The listing builds one solid part. Answer for the finished solid, in the listing's coordinates (mm). A direction names the side the tool comes from. Coordinates: 2 decimals unless noted, no trailing zeros. Loops run counter-clockwise (first coordinate to the right, second up) from the corner with the lowest first, then second, coordinate; pieces in that order, holes last. Notation, with made-up numbers: M 68.5,-14.75 L 87.5,-14.75 A27 cw 87.5,16.25 Z; hole C 11,-22 d1. An arc over 180 degrees is marked long. Answer as a JSON object with one key per item and string values. Group by question number.
1. A cutting plane is placed at B-B on z = 0. Give the vertices of the cut face in (x, y).
2. Straight lines are drawn through the part: L1, parallel to Z at x = 38.1, y = -8; L2, parallel to X at y = -13, z = -25; L3, parallel to Z at x = -42.5, y = -12.5. For each, find the intervals that lie inside material, in ascending order.
3. Given pin 1 (1.5 mm diameter, centred on x = -7, y = -22.5, fed in from -Z); pin 2 (6 mm diameter, centred on x = -20.5, y = -39.5, fed in from -Z); pin 3 (1 mm diameter, centred on y = -52, z = -3, fed in from +X); pin 4 (11.5 mm diameter, centred on x = -38.1, z = -25.4, fed in from -Y), each flat-ended and moving along its own axis, determine where each tip first touches the part or whether it passes through.
4. A cutting plane is placed at C-C on y = -12.5. Give the vertices of the cut face in (x, z), and give its area (3 significant figures).
5. Determine the mould class of faces 1 (the face through (-5.506, -26.871, 24.796)), 2 (the face through (33.06, -10.43, -29.26)), 3 (the face through (0, -58.674, 0)) for opening direction X: released by +X, released by -X, zero draft, split by the parting line, or undercut.
6. A cutting plane is placed at D-D on x = 0. Give the vertices of the cut face in (y, z).
7. For faces 4 (the face through (31, -20.574, 0)), 5 (the face through (17, -33.274, 9)), 6 (the face through (-32.234, -10.431, 22.968)), determine the directions among +Z, -Z, +X, -X, +Y, -Y from which every point of the face is accessible in a straight line to the end or side of a thin tool.
8. A cutting plane is placed at A-A on x = 38.1. Give the vertices of the cut face in (y, z).
from build123d import *

# Parameters (mm, degrees)
F0_W     = 101.6
F0_H     = 76.2
F1_DEPTH = 20.574
F2_R     = 6.35
F3_DEPTH = 25.4
F4_W     = 25.4
F4_H     = 38.1
F6_W     = 6.35
F6_H     = 14.2712268918
F8_SIZE  = 2.54
F9_R     = 2.54
F10_R    = 2.54


with BuildPart() as f1:
    # F0 (on Front) → F1 (new body)
    with BuildSketch(Plane.XZ):
        Rectangle(F0_W, F0_H)
    extrude(amount=F1_DEPTH)

    # F2 (on face) → F3 (cut)
    with BuildSketch(Plane.XZ.offset(20.574)):
        with Locations((38.1, -25.4)):
            Circle(F2_R)
        with Locations((-38.1, -25.4)):
            Circle(F2_R)
        with Locations((-38.1, 25.4)):
            Circle(F2_R)
        with Locations((38.1, 25.4)):
            Circle(F2_R)
    extrude(amount=-F3_DEPTH, mode=Mode.SUBTRACT)

    # F4 (on Top) → F5 (revolve)
    with BuildSketch(Plane.XY):
        with Locations((12.7, -39.624)):
            Rectangle(F4_W, F4_H)
    revolve(axis=Axis((0, -39.624, 0), (0, 1, 0)))

    # F6 (on Right) → F7 (revolve, cut)
    with BuildSketch(Plane.YZ):
        with Locations((-36.449, 26.1856134459)):
            Rectangle(F6_W, F6_H)
    revolve(axis=Axis((0, -58.674, 0), (0, 1, 0)), mode=Mode.SUBTRACT)

    # F8
    f8_edges = [f1.edges().sort_by_distance(p)[0] for p in [
        (0, -20.574, 38.1),
        (50.8, -20.574, 0),
        (0, -20.574, -38.1),
        (-50.8, -20.574, 0),
    ]]
    chamfer(f8_edges, length=F8_SIZE)

    # F9
    f9_edges = [f1.edges().sort_by_distance(p)[0] for p in [
        (-25.4, -20.574, 0),
        (-25.4, -33.274, 0),
        (-25.4, -39.624, 0),
    ]]
    fillet(f9_edges, radius=F9_R)

    # F10
    f10_edges = [f1.edges().sort_by_distance(p)[0] for p in [
        (-25.4, -58.674, 0),
    ]]
    fillet(f10_edges, radius=F10_R)


solid = f1.part
From the geometry:
{
 "1": {"outline": "M -50.8,-18.03 L -48.26,-20.57 L -27.94,-20.57 A2.54 cw -25.4,-23.11 L -25.4,-30.73 A2.54 ccw -22.86,-33.27 L -19.05,-33.27 L -19.05,-39.62 L -22.86,-39.62 A2.54 ccw -25.4,-42.16 L -25.4,-56.13 A2.54 ccw -22.86,-58.67 L 22.86,-58.67 A2.54 ccw 25.4,-56.13 L 25.4,-42.16 A2.54 ccw 22.86,-39.62 L 19.05,-39.62 L 19.05,-33.27 L 22.86,-33.27 A2.54 ccw 25.4,-30.73 L 25.4,-23.11 A2.54 cw 27.94,-20.57 L 48.26,-20.57 L 50.8,-18.03 L 50.8,0 L -50.8,0 Z"},
 "2": {"L1": "z = -38.1 to -31.75, -19.05 to 19.05, 31.75 to 38.1", "L2": "x = -50.8 to -44.44, -31.76 to 31.76, 44.44 to 50.8", "L3": "z = -38.1 to -29.98, -20.82 to 20.82, 29.98 to 38.1"},
 "3": {"pin 1": "stops at z = -24.87", "pin 2": "stops at z = -17.63", "pin 3": "stops at x = 25.28", "pin 4": "passes through"},
 "4": {"outline": "M -50.8,-38.1 L 50.8,-38.1 L 50.8,38.1 L -50.8,38.1 Z; hole C -38.1,-25.4 d12.7; hole C -38.1,25.4 d12.7; hole C 38.1,-25.4 d12.7; hole C 38.1,25.4 d12.7", "area": "7,240 mm²"},
 "5": {"face 1": "split by the parting line", "face 2": "undercut", "face 3": "zero draft"},
 "6": {"outline": "M -58.67,-22.86 A2.54 ccw -56.13,-25.4 L -42.16,-25.4 A2.54 ccw -39.62,-22.86 L -39.62,-19.05 L -33.27,-19.05 L -33.27,-22.86 A2.54 ccw -30.73,-25.4 L -23.11,-25.4 A2.54 cw -20.57,-27.94 L -20.57,-35.56 L -18.03,-38.1 L 0,-38.1 L 0,38.1 L -18.03,38.1 L -20.57,35.56 L -20.57,27.94 A2.54 cw -23.11,25.4 L -30.73,25.4 A2.54 ccw -33.27,22.86 L -33.27,19.05 L -39.62,19.05 L -39.62,22.86 A2.54 ccw -42.16,25.4 L -56.13,25.4 A2.54 ccw -58.67,22.86 Z"},
 "7": {"face 4": "-Y", "face 5": "none", "face 6": "+Y, -Y"},
 "8": {"outline": "M -20.57,-35.56 L -18.03,-38.1 L 0,-38.1 L 0,-31.75 L -20.57,-31.75 Z; M -20.57,-19.05 L 0,-19.05 L 0,19.05 L -20.57,19.05 Z; M -20.57,31.75 L 0,31.75 L 0,38.1 L -18.03,38.1 L -20.57,35.56 Z"}
}
